from build123d import *

# Parameters (mm, degrees)
SKETCH_1_W                         = 329
SKETCH_1_H                         = 193.5
SM_BASE_FLANGE_1_DEPTH             = 1.5
SM_EDGE_FLANGE_1_STRIP_W           = 7.4732
SM_EDGE_FLANGE_1_STRIP_H           = 1.5
SM_EDGE_FLANGE_1_STRIP_CUT_DEPTH   = 329
SM_EDGE_FLANGE_1_STRIP_2_W         = 7.4732
SM_EDGE_FLANGE_1_STRIP_2_H         = 1.5
SM_EDGE_FLANGE_1_STRIP_CUT_2_DEPTH = 329
SM_EDGE_FLANGE_1_DEPTH             = 329
SM_EDGE_FLANGE_1_BEND_DEPTH        = 329
SKETCH_21_R                        = 1.6
CUT_EXTRUDE_2_DEPTH                = 217


# Sheet-metal steps are written as plain solids
with BuildPart() as part:
    # Sketch 1 → Базовая кромка1 (new body)
    with BuildSketch(Plane(origin=(0, 0, 0), x_dir=(1, 0, 0), z_dir=(0, 1, 0))):
        with Locations((1.82103321, 33.150369004)):
            Rectangle(SKETCH_1_W, SKETCH_1_H)
    extrude(amount=-SM_BASE_FLANGE_1_DEPTH)

    # Ребро-кромка1 strip (across the edge) → Ребро-кромка1 strip cut (cut)
    with BuildSketch(Plane(origin=(166.32103321, 0, -129.900369004), x_dir=(0, 0, 1), z_dir=(-1, 0, 0))):
        with Locations((-1.5, -0.75)):
            Rectangle(SM_EDGE_FLANGE_1_STRIP_W, SM_EDGE_FLANGE_1_STRIP_H)
    extrude(amount=SM_EDGE_FLANGE_1_STRIP_CUT_DEPTH, mode=Mode.SUBTRACT)

    # Ребро-кромка1 strip 2 (across the edge) → Ребро-кромка1 strip cut 2 (cut)
    with BuildSketch(Plane(origin=(-162.67896679, 0, 63.599630996), x_dir=(0, 0, -1), z_dir=(1, 0, 0))):
        with Locations((-1.5, -0.75)):
            Rectangle(SM_EDGE_FLANGE_1_STRIP_2_W, SM_EDGE_FLANGE_1_STRIP_2_H)
    extrude(amount=SM_EDGE_FLANGE_1_STRIP_CUT_2_DEPTH, mode=Mode.SUBTRACT)

    # Ребро-кромка1 section (across the edge) → Ребро-кромка1 (add)
    with BuildSketch(Plane(origin=(166.32103321, 0, -129.900369004), x_dir=(0, 0, 1), z_dir=(-1, 0, 0))):
        with BuildLine():
            Line((0, 0.7366), (0, 194))
            Line((0, 194), (1.5, 194))
            Line((1.5, 194), (1.5, 0.7366))
            ThreePointArc((1.5, 0.7366), (1.715745145, 0.215745145), (2.2366, 0))
            Line((2.2366, 0), (2.2366, -1.5))
            ThreePointArc((2.2366, -1.5), (0.655084973, -0.844915027), (0, 0.7366))
        make_face()
    extrude(amount=SM_EDGE_FLANGE_1_DEPTH)

    # Ребро-кромка1 section 2 (across the edge) → Ребро-кромка1 bend (add)
    with BuildSketch(Plane(origin=(-162.67896679, 0, 63.599630996), x_dir=(0, 0, -1), z_dir=(1, 0, 0))):
        with BuildLine():
            Line((0, 0.7366), (0, 194))
            Line((0, 194), (1.5, 194))
            Line((1.5, 194), (1.5, 0.7366))
            ThreePointArc((1.5, 0.7366), (1.715745145, 0.215745145), (2.2366, 0))
            Line((2.2366, 0), (2.2366, -1.5))
            ThreePointArc((2.2366, -1.5), (0.655084973, -0.844915027), (0, 0.7366))
        make_face()
    extrude(amount=SM_EDGE_FLANGE_1_BEND_DEPTH)

    # Эскиз21 → Вырез-Вытянуть2 (cut)
    with BuildSketch(Plane(origin=(0, 0, -129.900369004), x_dir=(-1, 0, 0), z_dir=(0, 0, -1))):
        with Locations((-156.82103321, 12)):
            Circle(SKETCH_21_R)
        with Locations((-156.82103321, 54)):
            Circle(SKETCH_21_R)
        with Locations((-156.82103321, 96)):
            Circle(SKETCH_21_R)
        with Locations((-156.82103321, 138)):
            Circle(SKETCH_21_R)
        with Locations((-156.82103321, 180)):
            Circle(SKETCH_21_R)
        with Locations((153.17896679, 181.5)):
            Circle(SKETCH_21_R)
        with Locations((153.17896679, 139)):
            Circle(SKETCH_21_R)
        with Locations((153.17896679, 96.5)):
            Circle(SKETCH_21_R)
        with Locations((153.17896679, 54)):
            Circle(SKETCH_21_R)
        with Locations((153.17896679, 12)):
            Circle(SKETCH_21_R)
    extrude(amount=-CUT_EXTRUDE_2_DEPTH, mode=Mode.SUBTRACT)


solid = part.part
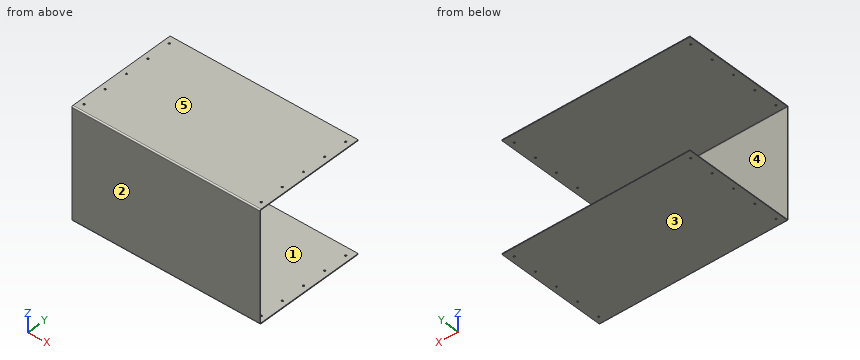
Part model, mm, in its own coordinate system. Face numbers are marked on the shaded views. A direction names the side the tool comes from. Give positions to 0.01 mm unless a question says otherwise; leave off trailing zeros. Order: outer loops, then holes, each group sorted by start corner. A loop starts at its lowest first (then second) coordinate and runs counter-clockwise, first axis right, second up. Notation, with made-up numbers: (23.25, -38) - (77.25, -38) arc R11 ccw to (77.25, -28) - close; hole circle Ø2 at (-13, -26.5). An arc over 180 degrees is marked (long way). Use a Markdown table: item, result.
1) Saw through at C-C on z = -20. List the corners of the cut face in (x, y).
Checked values:
| item | result |
|---|---|
| outline | (-162.68, -1.5) - (166.32, -1.5) - (166.32, 0) - (-162.68, 0) - close |
2) Probe L1, parallel to Z at x = 7.5, y = 154.5; L2, parallel to Y at x = -6, z = -93; L3, parallel to X at y = 139, z = -129.4. List the from-to ranges inside material, lowest first. Write a range as from..to.
Checked values:
| item | result |
|---|---|
| L1 | -129.9..-128.4, 62.1..63.6 |
| L2 | -1.5..0 |
| L3 | -162.68..-154.78, -151.58..155.57, 158.07..166.32 |
3) 3-axis set-ups, long thin cutter, end or side, ignore diameter. For the marked faces 4 and 5: which of +Z, -Z, +X, -X, +Y, -Y reach the whole face in a straight line?
Checked values:
| item | result |
|---|---|
| face 4 | +X, -X, +Y |
| face 5 | +Z, +X, -X, +Y, -Y |
4) Flat gauge pin, fed straight in: P1, Ø5, axis at x = 43.5, z = 32.5, coming from the +Y side. Where does the tip first touch, or does it go through?
Checked values:
| item | result |
|---|---|
| P1 | y = 0 |
5) Saw through at A-A on y = 129. List the corners of the cut face in (x, z).
Checked values:
| item | result |
|---|---|
| outline | (-162.68, -129.9) - (166.32, -129.9) - (166.32, -128.4) - (-162.68, -128.4) - close; (-162.68, 62.1) - (166.32, 62.1) - (166.32, 63.6) - (-162.68, 63.6) - close |
6) Two-plate mould, pull along Z, no slides. Class the marked faces 1, 2 and 3: +Z half, -Z half, draft (parallel to the pull), parting line (faces both ways), or undercut.
Checked values:
| item | result |
|---|---|
| face 1 | undercut |
| face 2 | draft |
| face 3 | -Z half |
7) Saw through at B-B on x = 63. List the corners of the cut face in (y, z), plus the area to 3 significant figures.
Checked values:
| item | result |
|---|---|
| outline | (-1.5, -127.66) arc R2.24 ccw to (0.74, -129.9) - (194, -129.9) - (194, -128.4) - (0.74, -128.4) arc R0.74 cw to (0, -127.66) - (0, 61.36) arc R0.74 cw to (0.74, 62.1) - (194, 62.1) - (194, 63.6) - (0.74, 63.6) arc R2.24 ccw to (-1.5, 61.36) - close |
| area | 870 mm² |
